from build123d import *

# Parameters (mm, degrees)
BASE_FLANGE1_DEPTH = 469.9
SKETCH10_W         = 152.4
SKETCH10_H         = 61.9125
CUT_EXTRUDE5_DEPTH = 510.278313523


# Sheet-metal steps are written as plain solids
with BuildPart() as part:
    # Sketch1 → Base-Flange1 (new body)
    with BuildSketch(Plane(origin=(0, 0, 0), x_dir=(0, 0, -1), z_dir=(1, 0, 0))):
        with BuildLine():
            Line((0, 0), (146.05, 0))
            ThreePointArc((146.05, 0), (150.540128061, 1.859871939), (152.4, 6.35))
            Line((152.4, 6.35), (152.4, 117.475))
            ThreePointArc((152.4, 117.475), (150.540128061, 121.965128061), (146.05, 123.825))
            Line((146.05, 123.825), (0, 123.825))
            Line((0, 123.825), (0, 120.65))
            Line((0, 120.65), (146.05, 120.65))
            ThreePointArc((146.05, 120.65), (148.29506403, 119.72006403), (149.225, 117.475))
            Line((149.225, 117.475), (149.225, 6.35))
            ThreePointArc((149.225, 6.35), (148.29506403, 4.10493597), (146.05, 3.175))
            Line((146.05, 3.175), (0, 3.175))
            Line((0, 3.175), (0, 0))
        make_face()
    extrude(amount=BASE_FLANGE1_DEPTH)

    # Sketch10 → Cut-Extrude5 (cut, through all)
    with BuildSketch(Plane(origin=(469.9, 0, 0), x_dir=(0, 0, -1), z_dir=(1, 0, 0))):
        with Locations((76.2, 30.95625)):
            Rectangle(SKETCH10_W, SKETCH10_H)
    extrude(amount=-CUT_EXTRUDE5_DEPTH, mode=Mode.SUBTRACT)


solid = part.part
Source: CAD feature listing. Evaluate the final solid. Frame: model axes, mm. A direction names the side the tool comes from. Give positions to 0.01 mm unless a question says otherwise; leave off trailing zeros. Order: outer loops, then holes, each group sorted by start corner. A loop starts at its lowest first (then second) coordinate and runs counter-clockwise, first axis right, second up. Notation, with made-up numbers: (-27, 18) -> (-6, 18) arc R12 cw to (-6, 27) -> close; hole circle Ø5 at (-1, 52). An arc over 180 degrees is marked (long way). Write item = value, one per line.
Q1. Cut plane B-B, the plane y = 113. Output: boundary loops of the cut face in (x, z) (3 decimals).
Data:
outline = (0, -152.4) -> (469.9, -152.4) -> (469.9, -149.225) -> (0, -149.225) -> close
Q2. Material intervals for line 1 (Z direction, x = 371.5, y = 80.5) (3 decimals); line 2 (Y direction, x = 428.5, z = -105) (3 decimals); line 3 (Z direction, x = 21, y = 121), sorted ascending. Write a range as from..to.
Data:
line_1 = -152.4..-149.225
line_2 = 120.65..123.825
line_3 = -151.33..0
Q3. Cut plane C-C, the plane z = -126. Output: boundary loops of the cut face in (x, y) (3 decimals), and give its area (3 significant figures).
Data:
outline = (0, 120.65) -> (469.9, 120.65) -> (469.9, 123.825) -> (0, 123.825) -> close
area = 1,490 mm^2
Q4. Set-up query: faces 1 (the face through (232, 120.65, -72)), 2 (the face through (232, 123.825, -74)). Return all of +Z, -Z, +X, -X, +Y, -Y with unobstructed straight access to the full face (end or side cutting, diameter ignored); none if empty.
Data:
face_1 = +Z, +X, -X, -Y
face_2 = +Z, -Z, +X, -X, +Y
Q5. Pin query (flat end, axial travel): pin 1 (12 mm diameter, centred on x = 354, y = 86, fed in from +Z) (3 decimals); pin 2 (5 mm diameter, centred on x = 189.5, z = -107, fed in from -Y). Return the tip coordinate at first contact, or that it passes through.
Data:
pin_1 = -149.225
pin_2 = 120.65
